CAD build for the part. Positions are in the model's coordinates, mm. Give positions to 0.01 mm unless a question says otherwise; leave off trailing zeros. Return JSON: item names as keys, results as strings.
from build123d import *

# Parameters (mm, degrees)
SKETCH1_R           = 3.4
BOSS_EXTRUDE1_DEPTH = 1500


with BuildPart() as part:
    # Sketch1 → Boss-Extrude1 (new body)
    with BuildSketch(Plane.XY):
        with BuildLine():
            Line((20, 17.75), (20, 5.15))
            Line((20, 5.15), (19, 5.15))
            Line((19, 5.15), (19, 4.15))
            Line((19, 4.15), (15.4, 4.15))
            Line((15.4, 4.15), (15.4, 6.35))
            Line((15.4, 6.35), (16.95, 6.35))
            ThreePointArc((16.95, 6.35), (17.833883476, 6.716116524), (18.2, 7.6))
            Line((18.2, 7.6), (18.2, 9.3))
            ThreePointArc((18.2, 9.3), (17.907106781, 10.007106781), (17.2, 10.3))
            Line((17.2, 10.3), (12.03669957, 10.3))
            ThreePointArc((12.03669957, 10.3), (11.73040037, 10.239040459), (11.470780817, 10.065452001))
            Line((11.470780817, 10.065452001), (6.084081247, 4.674305984))
            ThreePointArc((6.084081247, 4.674305984), (5.910833239, 4.414848262), (5.85, 4.108853983))
            Line((5.85, 4.108853983), (5.85, -4.108853983))
            ThreePointArc((5.85, -4.108853983), (5.910833239, -4.414848262), (6.084081247, -4.674305984))
            Line((6.084081247, -4.674305984), (11.470780817, -10.065452001))
            ThreePointArc((11.470780817, -10.065452001), (11.73040037, -10.239040459), (12.03669957, -10.3))
            Line((12.03669957, -10.3), (17.2, -10.3))
            ThreePointArc((17.2, -10.3), (17.907106781, -10.007106781), (18.2, -9.3))
            Line((18.2, -9.3), (18.2, -7.6))
            ThreePointArc((18.2, -7.6), (17.833883476, -6.716116524), (16.95, -6.35))
            Line((16.95, -6.35), (15.4, -6.35))
            Line((15.4, -6.35), (15.4, -4.15))
            Line((15.4, -4.15), (19, -4.15))
            Line((19, -4.15), (19, -5.15))
            Line((19, -5.15), (20, -5.15))
            Line((20, -5.15), (20, -17.75))
            ThreePointArc((20, -17.75), (19.340990258, -19.340990258), (17.75, -20))
            Line((17.75, -20), (5.15, -20))
            Line((5.15, -20), (5.15, -19))
            Line((5.15, -19), (4.15, -19))
            Line((4.15, -19), (4.15, -15.4))
            Line((4.15, -15.4), (6.35, -15.4))
            Line((6.35, -15.4), (6.35, -16.95))
            ThreePointArc((6.35, -16.95), (6.716116524, -17.833883476), (7.6, -18.2))
            Line((7.6, -18.2), (9.3, -18.2))
            ThreePointArc((9.3, -18.2), (10.007106781, -17.907106781), (10.3, -17.2))
            Line((10.3, -17.2), (10.3, -12.054477022))
            ThreePointArc((10.3, -12.054477022), (10.239166761, -11.748482743), (10.065918753, -11.489025021))
            Line((10.065918753, -11.489025021), (4.665899173, -6.084547999))
            ThreePointArc((4.665899173, -6.084547999), (4.406279619, -5.910959541), (4.09998042, -5.85))
            Line((4.09998042, -5.85), (-4.09998042, -5.85))
            ThreePointArc((-4.09998042, -5.85), (-4.406279619, -5.910959541), (-4.665899173, -6.084547999))
            Line((-4.665899173, -6.084547999), (-10.065918753, -11.489025021))
            ThreePointArc((-10.065918753, -11.489025021), (-10.239166761, -11.748482743), (-10.3, -12.054477022))
            Line((-10.3, -12.054477022), (-10.3, -17.2))
            ThreePointArc((-10.3, -17.2), (-10.007106781, -17.907106781), (-9.3, -18.2))
            Line((-9.3, -18.2), (-7.6, -18.2))
            ThreePointArc((-7.6, -18.2), (-6.716116524, -17.833883476), (-6.35, -16.95))
            Line((-6.35, -16.95), (-6.35, -15.4))
            Line((-6.35, -15.4), (-4.15, -15.4))
            Line((-4.15, -15.4), (-4.15, -19))
            Line((-4.15, -19), (-5.15, -19))
            Line((-5.15, -19), (-5.15, -20))
            Line((-5.15, -20), (-17.75, -20))
            ThreePointArc((-17.75, -20), (-19.340990258, -19.340990258), (-20, -17.75))
            Line((-20, -17.75), (-20, -5.15))
            Line((-20, -5.15), (-19, -5.15))
            Line((-19, -5.15), (-19, -4.15))
            Line((-19, -4.15), (-15.4, -4.15))
            Line((-15.4, -4.15), (-15.4, -6.35))
            Line((-15.4, -6.35), (-16.95, -6.35))
            ThreePointArc((-16.95, -6.35), (-17.833883476, -6.716116524), (-18.2, -7.6))
            Line((-18.2, -7.6), (-18.2, -9.3))
            ThreePointArc((-18.2, -9.3), (-17.907106781, -10.007106781), (-17.2, -10.3))
            Line((-17.2, -10.3), (-12.03669957, -10.3))
            ThreePointArc((-12.03669957, -10.3), (-11.73040037, -10.239040459), (-11.470780817, -10.065452001))
            Line((-11.470780817, -10.065452001), (-6.084081247, -4.674305984))
            ThreePointArc((-6.084081247, -4.674305984), (-5.910833239, -4.414848262), (-5.85, -4.108853983))
            Line((-5.85, -4.108853983), (-5.85, 4.108853983))
            ThreePointArc((-5.85, 4.108853983), (-5.910833239, 4.414848262), (-6.084081247, 4.674305984))
            Line((-6.084081247, 4.674305984), (-11.470780817, 10.065452001))
            ThreePointArc((-11.470780817, 10.065452001), (-11.73040037, 10.239040459), (-12.03669957, 10.3))
            Line((-12.03669957, 10.3), (-17.2, 10.3))
            ThreePointArc((-17.2, 10.3), (-17.907106781, 10.007106781), (-18.2, 9.3))
            Line((-18.2, 9.3), (-18.2, 7.6))
            ThreePointArc((-18.2, 7.6), (-17.833883476, 6.716116524), (-16.95, 6.35))
            Line((-16.95, 6.35), (-15.4, 6.35))
            Line((-15.4, 6.35), (-15.4, 4.15))
            Line((-15.4, 4.15), (-19, 4.15))
            Line((-19, 4.15), (-19, 5.15))
            Line((-19, 5.15), (-20, 5.15))
            Line((-20, 5.15), (-20, 17.75))
            ThreePointArc((-20, 17.75), (-19.340990258, 19.340990258), (-17.75, 20))
            Line((-17.75, 20), (-5.15, 20))
            Line((-5.15, 20), (-5.15, 19))
            Line((-5.15, 19), (-4.15, 19))
            Line((-4.15, 19), (-4.15, 15.4))
            Line((-4.15, 15.4), (-6.35, 15.4))
            Line((-6.35, 15.4), (-6.35, 16.95))
            ThreePointArc((-6.35, 16.95), (-6.716116524, 17.833883476), (-7.6, 18.2))
            Line((-7.6, 18.2), (-9.3, 18.2))
            ThreePointArc((-9.3, 18.2), (-10.007106781, 17.907106781), (-10.3, 17.2))
            Line((-10.3, 17.2), (-10.3, 12.054477022))
            ThreePointArc((-10.3, 12.054477022), (-10.239166761, 11.748482743), (-10.065918753, 11.489025021))
            Line((-10.065918753, 11.489025021), (-4.665899173, 6.084547999))
            ThreePointArc((-4.665899173, 6.084547999), (-4.406279619, 5.910959541), (-4.09998042, 5.85))
            Line((-4.09998042, 5.85), (4.09998042, 5.85))
            ThreePointArc((4.09998042, 5.85), (4.406279619, 5.910959541), (4.665899173, 6.084547999))
            Line((4.665899173, 6.084547999), (10.065918753, 11.489025021))
            ThreePointArc((10.065918753, 11.489025021), (10.239166761, 11.748482743), (10.3, 12.054477022))
            Line((10.3, 12.054477022), (10.3, 17.2))
            ThreePointArc((10.3, 17.2), (10.007106781, 17.907106781), (9.3, 18.2))
            Line((9.3, 18.2), (7.6, 18.2))
            ThreePointArc((7.6, 18.2), (6.716116524, 17.833883476), (6.35, 16.95))
            Line((6.35, 16.95), (6.35, 15.4))
            Line((6.35, 15.4), (4.15, 15.4))
            Line((4.15, 15.4), (4.15, 19))
            Line((4.15, 19), (5.15, 19))
            Line((5.15, 19), (5.15, 20))
            Line((5.15, 20), (17.75, 20))
            ThreePointArc((17.75, 20), (19.340990258, 19.340990258), (20, 17.75))
        make_face()
        Circle(SKETCH1_R, mode=Mode.SUBTRACT)
        with BuildLine():
            Line((18.6, 16.35), (18.6, 12.2))
            ThreePointArc((18.6, 12.2), (18.365685425, 11.634314575), (17.8, 11.4))
            Line((17.8, 11.4), (12.2, 11.4))
            ThreePointArc((12.2, 11.4), (11.634314575, 11.634314575), (11.4, 12.2))
            Line((11.4, 12.2), (11.4, 17.8))
            ThreePointArc((11.4, 17.8), (11.634314575, 18.365685425), (12.2, 18.6))
            Line((12.2, 18.6), (16.35, 18.6))
            ThreePointArc((16.35, 18.6), (17.940990258, 17.940990258), (18.6, 16.35))
        make_face(mode=Mode.SUBTRACT)
        with BuildLine():
            Line((-12.2, 18.6), (-16.35, 18.6))
            ThreePointArc((-16.35, 18.6), (-17.940990258, 17.940990258), (-18.6, 16.35))
            Line((-18.6, 16.35), (-18.6, 12.2))
            ThreePointArc((-18.6, 12.2), (-18.365685425, 11.634314575), (-17.8, 11.4))
            Line((-17.8, 11.4), (-12.2, 11.4))
            ThreePointArc((-12.2, 11.4), (-11.634314575, 11.634314575), (-11.4, 12.2))
            Line((-11.4, 12.2), (-11.4, 17.8))
            ThreePointArc((-11.4, 17.8), (-11.634314575, 18.365685425), (-12.2, 18.6))
        make_face(mode=Mode.SUBTRACT)
        with BuildLine():
            Line((-18.6, -16.35), (-18.6, -12.2))
            ThreePointArc((-18.6, -12.2), (-18.365685425, -11.634314575), (-17.8, -11.4))
            Line((-17.8, -11.4), (-12.2, -11.4))
            ThreePointArc((-12.2, -11.4), (-11.634314575, -11.634314575), (-11.4, -12.2))
            Line((-11.4, -12.2), (-11.4, -17.8))
            ThreePointArc((-11.4, -17.8), (-11.634314575, -18.365685425), (-12.2, -18.6))
            Line((-12.2, -18.6), (-16.35, -18.6))
            ThreePointArc((-16.35, -18.6), (-17.940990258, -17.940990258), (-18.6, -16.35))
        make_face(mode=Mode.SUBTRACT)
        with BuildLine():
            Line((12.2, -18.6), (16.35, -18.6))
            ThreePointArc((16.35, -18.6), (17.940990258, -17.940990258), (18.6, -16.35))
            Line((18.6, -16.35), (18.6, -12.2))
            ThreePointArc((18.6, -12.2), (18.365685425, -11.634314575), (17.8, -11.4))
            Line((17.8, -11.4), (12.2, -11.4))
            ThreePointArc((12.2, -11.4), (11.634314575, -11.634314575), (11.4, -12.2))
            Line((11.4, -12.2), (11.4, -17.8))
            ThreePointArc((11.4, -17.8), (11.634314575, -18.365685425), (12.2, -18.6))
        make_face(mode=Mode.SUBTRACT)
    extrude(amount=BOSS_EXTRUDE1_DEPTH)


solid = part.part
1. Cut at A-A, the plane z = 1410. Give the number of separate pieces and of enclosed holes in the cut face, plus the area to 3 significant figures.
Values follow:
{"separate pieces": "1", "enclosed holes": "5", "area": "464 mm²"}
2. Drill centre lines: probe 1 along Y at (x, z) = (-17, 737); probe 2 along Y at (x, z) = (15, 257.5); probe 3 along X at (y, z) = (11.5, 173.5). Where is each one in solid material? Low to high.
Values follow:
{"probe 1": "y = -20 to -18.5, -11.4 to -10.3, -6.35 to -4.15, 4.15 to 6.35, 10.3 to 11.4, 18.5 to 20", "probe 2": "y = -20 to -18.6, -11.4 to -10.3, 10.3 to 11.4, 18.6 to 20", "probe 3": "x = -20 to -18.19, -11.81 to -10.08, 10.08 to 11.81, 18.19 to 20"}
3. Drop flat-ended pins along their axis: P1, Ø0.5, axis at y = 4.5, z = 814.5, coming from the +X side; P2, Ø0.5, axis at x = -4.5, z = 676.5, coming from the -Y side; P3, Ø2.5, axis at x = -2, z = 682.5, coming from the +Y side. Give the stop position or say it passes through.
Values follow:
{"P1": "stops at x = 19", "P2": "stops at y = -19", "P3": "stops at y = 5.85"}
